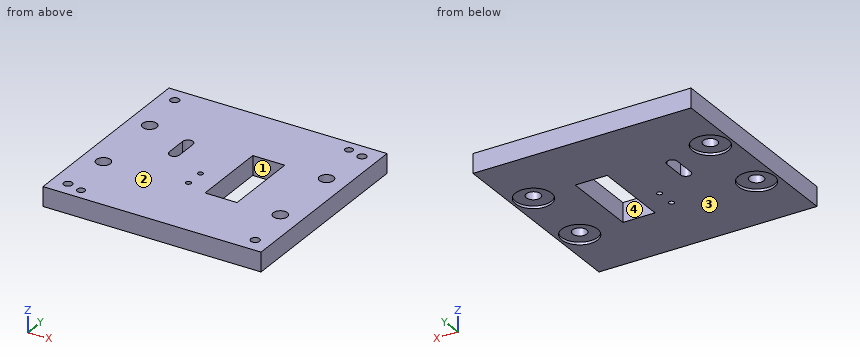
from build123d import *

# Parameters (mm, degrees)
SKETCH2_W                           = 169.5
SKETCH2_H                           = 158
SKETCH2_R                           = 2
SKETCH2_W_2                         = 24.88
SKETCH2_H_2                         = 59.88
BOSS_EXTRUDE1_DEPTH                 = 15
M8X1_25_TAPPED_HOLE1_D              = 6.8
M8X1_25_TAPPED_HOLE1_DEPTH          = 7.5
M8X1_25_TAPPED_HOLE1_TIP            = 2.042926105
F_6_0MM_CLEARANCE_DOWEL_HOLE1_D     = 6
F_6_0MM_CLEARANCE_DOWEL_HOLE1_DEPTH = 10
SKETCH7_R                           = 14
CUT_EXTRUDE1_DEPTH                  = 2
M10_CLEARANCE_HOLE1_D               = 11


with BuildPart() as part:
    # Sketch2 → Boss-Extrude1 (new body)
    with BuildSketch(Plane.XY):
        with Locations((34.75, 0)):
            Rectangle(SKETCH2_W, SKETCH2_H)
        with Locations((29, -9)):
            Circle(SKETCH2_R, mode=Mode.SUBTRACT)
        with Locations((29, -24)):
            Circle(SKETCH2_R, mode=Mode.SUBTRACT)
        with BuildLine():
            Line((-4, 22), (-4, 5))
            ThreePointArc((-4, 5), (0, 1), (4, 5))
            Line((4, 5), (4, 22))
            ThreePointArc((4, 22), (0, 26), (-4, 22))
        make_face(mode=Mode.SUBTRACT)
        with Locations((58, 0)):
            Rectangle(SKETCH2_W_2, SKETCH2_H_2, mode=Mode.SUBTRACT)
    extrude(amount=-BOSS_EXTRUDE1_DEPTH)

    # M8x1.25 Tapped Hole1
    with Locations(Plane(origin=(0, 0, 0), x_dir=(0.9063077870366375, -0.42261826174072625, 0), z_dir=(0, 0, 1))):
        with Locations((125.743510643, -15.291158594), (69.11266357, 106.154084869), (-62.755119444, 44.663127785), (-6.124272371, -76.782115678)):
            Hole(M8X1_25_TAPPED_HOLE1_D / 2, depth=M8X1_25_TAPPED_HOLE1_DEPTH)
            with Locations((0, 0, -(M8X1_25_TAPPED_HOLE1_DEPTH + M8X1_25_TAPPED_HOLE1_TIP / 2))):  # 118° drill point
                Cone(0, M8X1_25_TAPPED_HOLE1_D / 2, M8X1_25_TAPPED_HOLE1_TIP, mode=Mode.SUBTRACT)

    # Ø6.0mm Clearance Dowel Hole1
    with Locations(Plane(origin=(0, 0, 0), x_dir=(0.9063077870366375, -0.42261826174072625, 0), z_dir=(0, 0, 1))):
        with Locations((56.96911534, 103.801589089), (6.019275859, -74.429619898)):
            Hole(F_6_0MM_CLEARANCE_DOWEL_HOLE1_D / 2, depth=F_6_0MM_CLEARANCE_DOWEL_HOLE1_DEPTH)

    # Sketch7 → Cut-Extrude1 (cut)
    with BuildSketch(Plane(origin=(0, 0, -15), x_dir=(-1, 0, 0), z_dir=(0, 0, -1))):
        with Locations((-103.5, 29)):
            Circle(SKETCH7_R)
        with Locations((34, 29)):
            Circle(SKETCH7_R)
        with Locations((34, -29)):
            Circle(SKETCH7_R)
        with Locations((-103.5, -29)):
            Circle(SKETCH7_R)
    extrude(amount=-CUT_EXTRUDE1_DEPTH, mode=Mode.SUBTRACT)

    # M10 Clearance Hole1 (through all)
    with Locations(Plane(origin=(0, 0, 0), x_dir=(0.9063077870366375, -0.42261826174072625, 0), z_dir=(0, 0, 1))):
        with Locations((-43.07039435, 11.913904925), (-18.558535169, -40.651946723), (81.546926368, 70.023915914), (106.058785549, 17.458064266)):
            Hole(M10_CLEARANCE_HOLE1_D / 2)


solid = part.part
Design review of the part built by this model. Coordinates are the model's own, in mm. Face numbers are marked on the shaded views. A direction names the side the tool comes from. Give positions to 0.01 mm unless a question says otherwise; leave off trailing zeros. Order: outer loops, then holes, each group sorted by start corner. A loop starts at its lowest first (then second) coordinate and runs counter-clockwise, first axis right, second up. Notation, with made-up numbers: (-28, 28.25) - (23, 28.25) arc R17 cw to (23, 39.25) - close; hole circle Ø8 at (88, 35.5). An arc over 180 degrees is marked (long way). Write item = value, one per line. Start each with the question number.
Q1. Mouldability with a two-part tool opening along X and no side actions: class the marked faces 1 and 2 as released by +X, released by -X, zero draft, split by the parting line, or undercut.
Q2. We need section C-C on x = -2. State the section outline as (y, z) points, plus the area to 3 significant figures.
Q3. We need section D-D on x = -26. State the section outline as (y, z) points.
Q4. We need section A-A on x = 54. State the section outline as (y, z) points, plus the area to 3 significant figures.
Q5. To check wall thickness, follow L1, parallel to X at y = 11, z = -3; L2, parallel to Y at x = -34, z = -13.95; L3, parallel to X at y = 30.5, z = -10.5. State the ranges of each line that lie inside material, in increasing order. Write a range as from..to.
Q6. Clearance check with a flat-ended pin moving along its axis: pin 1 Ø8.5 at (x, y) = (-28, -25.5) entering from -Z. State where the tip first meets the part, or that it passes through.
Q7. We need section B-B on z = -3.25. State how many separate pieces and enclosed holes the cut face has, plus the area to 3 significant figures.
Q8. Tool access review of the marked faces 3 and 4: name each direction out of +Z, -Z, +X, -X, +Y, -Y from which nothing blocks a thin tool from reaching the whole face with its end or side.
Working result:
q1.face_1 = undercut
q1.face_2 = zero draft
q2.outline = (-79, -15) - (1.54, -15) - (1.54, 0) - (-79, 0) - close; (25.46, -15) - (79, -15) - (79, 0) - (25.46, 0) - close
q2.area = 2,010 mm²
q3.outline = (-79, -15) - (-40.49, -15) - (-40.49, -13) - (-17.51, -13) - (-17.51, -15) - (17.51, -15) - (17.51, -13) - (40.49, -13) - (40.49, -15) - (79, -15) - (79, 0) - (-67, 0) - (-67, -10) - (-73, -10) - (-73, 0) - (-79, 0) - close
q4.outline = (-79, -15) - (-29.94, -15) - (-29.94, 0) - (-79, 0) - close; (29.94, -15) - (79, -15) - (79, 0) - (29.94, 0) - close
q4.area = 1,470 mm²
q5.L1 = -50..-4, 4..45.56, 70.44..119.5
q5.L2 = -79..-43, -15..15, 43..79
q5.L3 = -50..-39.29, -28.71..98.21, 108.79..119.5
q6.pin_1 = -13
q7.separate_pieces = 1
q7.enclosed_holes = 14
q7.area = 24,500 mm²
q8.face_3 = -Z, +X, -X, +Y, -Y
q8.face_4 = +Z, -Z
